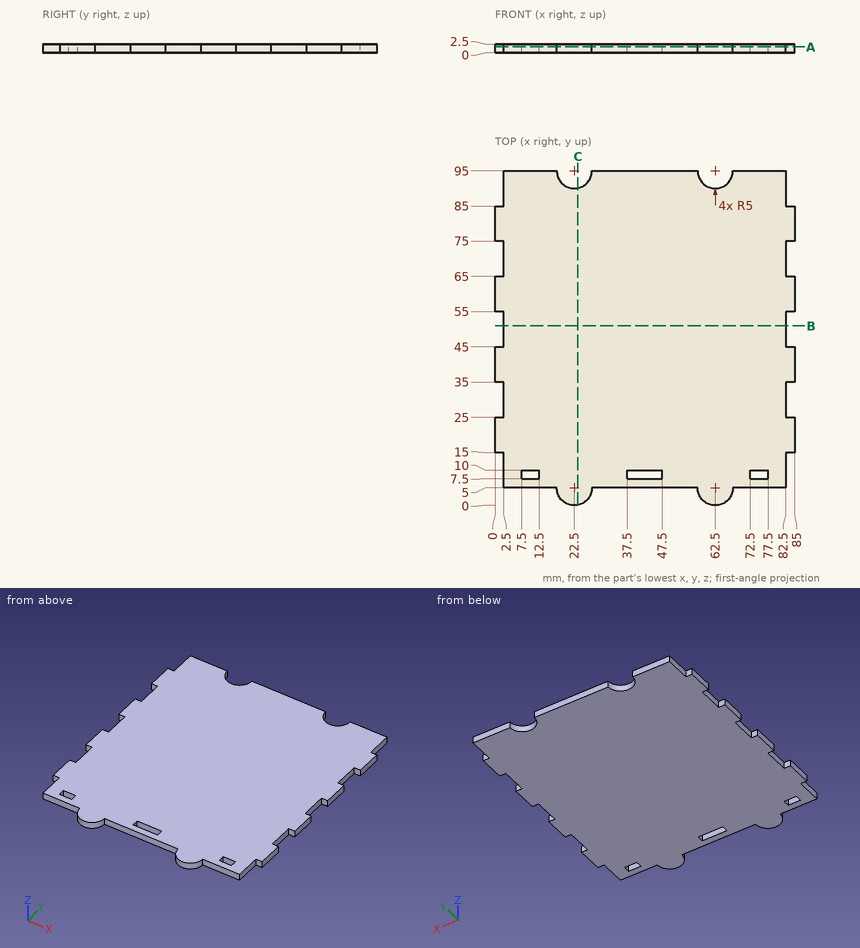
For this review, use the dimensioned drawing (mm, ordinates from the lowest corner) and the shaded views. Give positions to 0.01 mm unless a question says otherwise; leave off trailing zeros. Write each loop counter-clockwise with the first axis right and the second up, starting at its lowest first coordinate (ties: lowest second). Pieces come first, ordered by that corner, then holes. Notation, with made-up numbers: M 67,81.25 L 115,81.25 A22 ccw 115,118.25 Z; hole C -25.75,89.5 d7. An arc over 180 degrees is marked long. Write item = value, one per line. Start each with the question number.
Q1. For line 1 (Y direction, x = 77, z = 1.3); line 2 (Y direction, x = 4, z = 1.15); line 3 (X direction, y = 6.5, z = 0.3), list the stretches that pass through material, from the lowest coordinate up.
Q2. Clearance check with flat-ended pins moving along their axes: pin 1 (6 mm diameter, centred on x = 22, y = 58, fed in from -Z); pin 2 (0.8 mm diameter, centred on y = 30, z = 1, fed in from -X); pin 3 (1.2 mm diameter, centred on x = 83.5, z = 0.5, fed in from +Y); pin 4 (0.8 mm diameter, centred on x = 83, z = 1, fed in from -Y). State where each tip first meets the part, or that it passes through.
Q3. We need section A-A (z = 1.65). Give the number of separate pieces and of enclosed holes in the cut face, plus the area to 3 significant figures.
Q4. We need section C-C (x = 23.5). State the section outline as (y, z) points, plus the area to 3 significant figures.
Q5. We need section B-B (y = 51). State the section outline as (x, z) points, plus the area to 3 significant figures.
Result set:
q1.line_1 = 5 to 7.5, 10 to 95
q1.line_2 = 5 to 95
q1.line_3 = 2.5 to 82.5
q2.pin_1 = 0
q2.pin_2 = 2.5
q2.pin_3 = 85
q2.pin_4 = 15
q3.separate_pieces = 1
q3.enclosed_holes = 3
q3.area = 7,350 mm2
q4.outline = M 0.1,0 L 90.1,0 L 90.1,2.5 L 0.1,2.5 Z
q4.area = 225 mm2
q5.outline = M 2.5,0 L 82.5,0 L 82.5,2.5 L 2.5,2.5 Z
q5.area = 200 mm2
